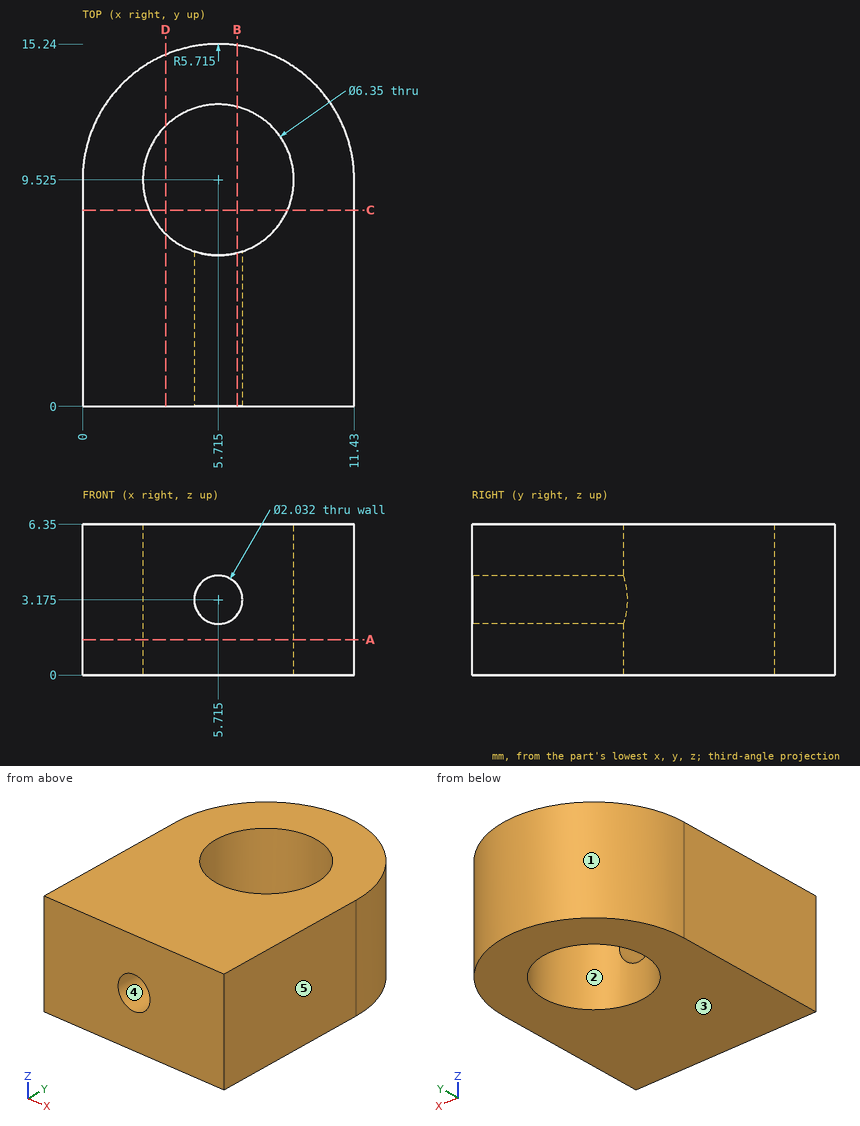
Drawing for the job (mm, zero at the part's lowest x, y, z). A direction names the side the tool comes from. Round coordinates to 2 decimals unless told otherwise and drop trailing zeros. Write each loop counter-clockwise with the first axis right and the second up, starting at its lowest first coordinate (ties: lowest second). Pieces come first, ordered by that corner, then holes. Notation, with made-up numbers: (56.25, -19.75) - (73.25, -19.75) arc R26 cw to (73.25, 12.25) - close; hole circle Ø11 at (-35.75, 68). An arc over 180 degrees is marked (long way). Write item = value, one per line. Start each with the question number.
Q1. Which spindle directions (+Z, -Z, +X, -X, +Y, -Y) get a long thin tool onto all of the face, cutting with end or side? Do the marked faces 4 and 5. Say none if no direction does.
Q2. Mould opens along Y. For the marked faces 1, 2 and 3 say: pulls with the +Y half, pulls with the -Y half, needs draft (parallel to the pull), parting line crosses it, or undercut.
Q3. Band-saw the part on C-C (y = 8.25). Give the cut face in (x, z).
Q4. Probe L1, parallel to X at y = 6, z = 3.25; L2, parallel to Z at x = 5, y = 1.25; L3, parallel to X at y = 11, z = 0.5. List the from-to ranges inside material, lowest first. Write a range as from..to.
Q5. Band-saw the part on D-D (x = 3.5). Give the cut face in (y, z), then the cut area to 3 significant figures.
Q6. Drop flat-ended pins along their axis: pin 1 (3 mm diameter, centred on x = 2, z = 4, fed in from +Y); pin 2 (2.5 mm diameter, centred on x = 5.715, z = 3.175, fed in from -Y); pin 3 (1.5 mm diameter, centred on y = 11, z = 4, fed in from +X). Give the stop position or say it passes through.
Q7. Band-saw the part on B-B (x = 6.5). Give the cut face in (y, z).
Q8. Band-saw the part on A-A (z = 1.5). Give the cut face in (x, y) (3 decimals), then the cut area to 3 significant figures.
Answers below:
q1.face_4 = -Y
q1.face_5 = +Z, -Z, +X, +Y, -Y
q2.face_1 = pulls with the +Y half
q2.face_2 = undercut
q2.face_3 = needs draft
q3.outline = (0, 0) - (2.81, 0) - (2.81, 6.35) - (0, 6.35) - close; (8.62, 0) - (11.43, 0) - (11.43, 6.35) - (8.62, 6.35) - close
q4.L1 = 0..4.7, 6.73..11.43
q4.L2 = 0..2.45, 3.9..6.35
q4.L3 = 0.19..2.9, 8.53..11.24
q5.outline = (0, 0) - (7.25, 0) - (7.25, 6.35) - (0, 6.35) - close; (11.8, 0) - (14.79, 0) - (14.79, 6.35) - (11.8, 6.35) - close
q5.area = 65.0 mm2
q6.pin_1 = 14.79
q6.pin_2 = 0
q6.pin_3 = 11.38
q7.outline = (0, 0) - (6.45, 0) - (6.45, 2.53) - (0, 2.53) - close; (0, 3.82) - (6.45, 3.82) - (6.45, 6.35) - (0, 6.35) - close; (12.6, 0) - (15.19, 0) - (15.19, 6.35) - (12.6, 6.35) - close
q8.outline = (0, 0) - (11.43, 0) - (11.43, 9.525) arc R5.715 ccw to (0, 9.525) - close; hole circle Ø6.35 at (5.715, 9.525)
q8.area = 129 mm2
